Here's how the part is built. I have some questions about the finished solid (model axes, mm). Round coordinates to 2 decimals unless told otherwise and drop trailing zeros. Write each loop counter-clockwise with the first axis right and the second up, starting at its lowest first coordinate (ties: lowest second). Pieces come first, ordered by that corner, then holes. Notation, with made-up numbers: (-7, 35) - (10, 35) arc R18 ccw to (10, 62) - close; hole circle Ø9 at (89, 67.5). An arc over 180 degrees is marked (long way). One line per item, written item: value. Start each with the question number.
Item 1: Imagine slicing it at A-A, the plane x = 139.6. Please give me the cut outline in (y, z).
Item 2: Imagine slicing it at B-B, the plane x = 67. Please give me the cut outline in (y, z).
Item 3: If I drill on line 1 (X direction, y = 81, z = 1.55); line 2 (X direction, y = 133, z = 1.7); line 3 (Y direction, x = 129.4, z = 0.8), over which ranges is the centre line in solid material (lowest first)?
Item 4: Imagine slicing it at C-C, the plane z = 1.7. Count the separate pieces of the cut face and the enclosed holes in it, then the cut area to 3 significant figures.
Item 5: Imagine slicing it at D-D, the plane y = 48. Please give me the cut outline in (x, z).
Item 6: For P1, Ø0.9, axis at y = 107.5, z = 1, coming from the -X side; P2, Ø1.8, axis at x = 61, y = 6, coming from the +Z side; P3, Ø1, axis at y = 48.5, z = 1.5, coming from the -X side, each with a flat end and sliding along its axis, tell me the tip position at first contact or that it passes through.
```python
from build123d import *

# Parameters (mm, degrees)
SKETCH_R   = 10.5
SKETCH_R_2 = 1.5
SKETCH_R_3 = 2
PAD_DEPTH  = 3


with BuildPart() as part:
    # Sketch → Pad (new body)
    with BuildSketch(Plane.XY):
        with BuildLine():
            Line((0, 0), (0, 24))
            Line((0, 24), (20, 24))
            Line((20, 24), (20, 39.85))
            Line((20, 39.85), (73, 39.85))
            Line((73, 39.85), (73, 84.15))
            Line((73, 84.15), (20, 84.15))
            Line((20, 84.15), (20, 100))
            Line((20, 100), (0, 100))
            Line((0, 100), (0, 160))
            Line((0, 160), (32, 160))
            Line((32, 160), (32, 120))
            Line((52, 120), (32, 120))
            Line((52, 100), (52, 120))
            Line((52, 100), (90, 100))
            Line((90, 100), (90, 34))
            ThreePointArc((90, 34), (75.857864, 28.142136), (70, 14))
            Line((70, 0), (70, 14))
            Line((0, 0), (70, 0))
        make_face()
        with Locations((16, 144)):
            Circle(SKETCH_R, mode=Mode.SUBTRACT)
        with Locations((22.3, 154.91192)):
            Circle(SKETCH_R_2, mode=Mode.SUBTRACT)
        with Locations((22.3, 133.08808)):
            Circle(SKETCH_R_2, mode=Mode.SUBTRACT)
        with Locations((3.4, 144)):
            Circle(SKETCH_R_2, mode=Mode.SUBTRACT)
        with Locations((30.2, 30.85)):
            Circle(SKETCH_R_3, mode=Mode.SUBTRACT)
        with Locations((40.4, 30.85)):
            Circle(SKETCH_R_3, mode=Mode.SUBTRACT)
        with Locations((50.6, 30.85)):
            Circle(SKETCH_R_3, mode=Mode.SUBTRACT)
        with Locations((60.8, 30.85)):
            Circle(SKETCH_R_3, mode=Mode.SUBTRACT)
        with Locations((30.2, 93.15)):
            Circle(SKETCH_R_3, mode=Mode.SUBTRACT)
        with Locations((40.4, 93.15)):
            Circle(SKETCH_R_3, mode=Mode.SUBTRACT)
        with Locations((50.6, 93.15)):
            Circle(SKETCH_R_3, mode=Mode.SUBTRACT)
        with Locations((60.8, 93.15)):
            Circle(SKETCH_R_3, mode=Mode.SUBTRACT)
        with Locations((76.5, 81)):
            Circle(SKETCH_R_2, mode=Mode.SUBTRACT)
        with Locations((76.5, 67)):
            Circle(SKETCH_R_2, mode=Mode.SUBTRACT)
        with Locations((61, 19)):
            Circle(SKETCH_R_2, mode=Mode.SUBTRACT)
        with Locations((61, 6)):
            Circle(SKETCH_R_2, mode=Mode.SUBTRACT)
        with Locations((8, 8)):
            Circle(SKETCH_R_2, mode=Mode.SUBTRACT)
        with Locations((86, 90)):
            Circle(SKETCH_R_2, mode=Mode.SUBTRACT)
        with Locations((16, 126.8)):
            Circle(SKETCH_R_2, mode=Mode.SUBTRACT)
        with Locations((16, 120.4)):
            Circle(SKETCH_R_2, mode=Mode.SUBTRACT)
    pad = extrude(amount=PAD_DEPTH)

    # Mirrored: Pad across face of Pad
    add(pad.mirror(Plane(origin=(90, 67, 1.5), x_dir=(0, 1, 0), z_dir=(1, 0, 0))))


solid = part.part
```
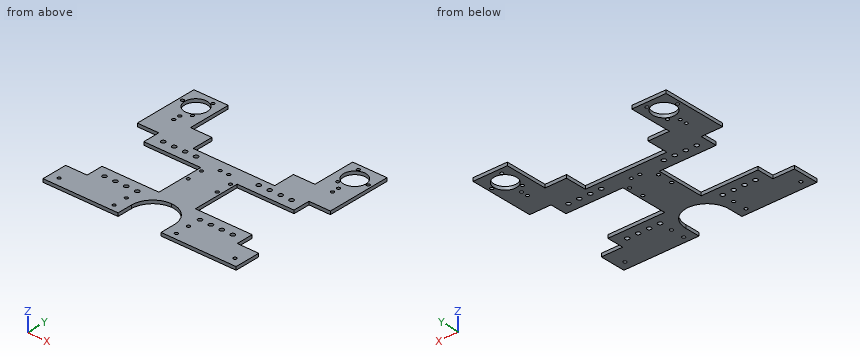
Values follow:
1. outline: (0, 0) - (28.85, 0) - (28.85, 3) - (0, 3) - close; (32.85, 0) - (39.85, 0) - (39.85, 3) - (32.85, 3) - close; (84.15, 0) - (91.15, 0) - (91.15, 3) - (84.15, 3) - close; (95.15, 0) - (120, 0) - (120, 3) - (95.15, 3) - close
2. outline: (0, 0) - (39.85, 0) - (39.85, 3) - (0, 3) - close; (84.15, 0) - (100, 0) - (100, 3) - (84.15, 3) - close
3. line 1: x = 73 to 75, 78 to 102, 105 to 107
3. line 2: x = 0 to 20.8, 23.8 to 32, 148 to 156.2, 159.2 to 180
3. line 3: y = 0 to 28.85, 32.85 to 39.85, 84.15 to 91.15, 95.15 to 120
4. separate pieces: 1
4. enclosed holes: 40
4. area: 12,700 mm^2
5. outline: (73, 0) - (107, 0) - (107, 3) - (73, 3) - close
6. P1: stops at x = 0
6. P2: passes through
6. P3: stops at x = 73
